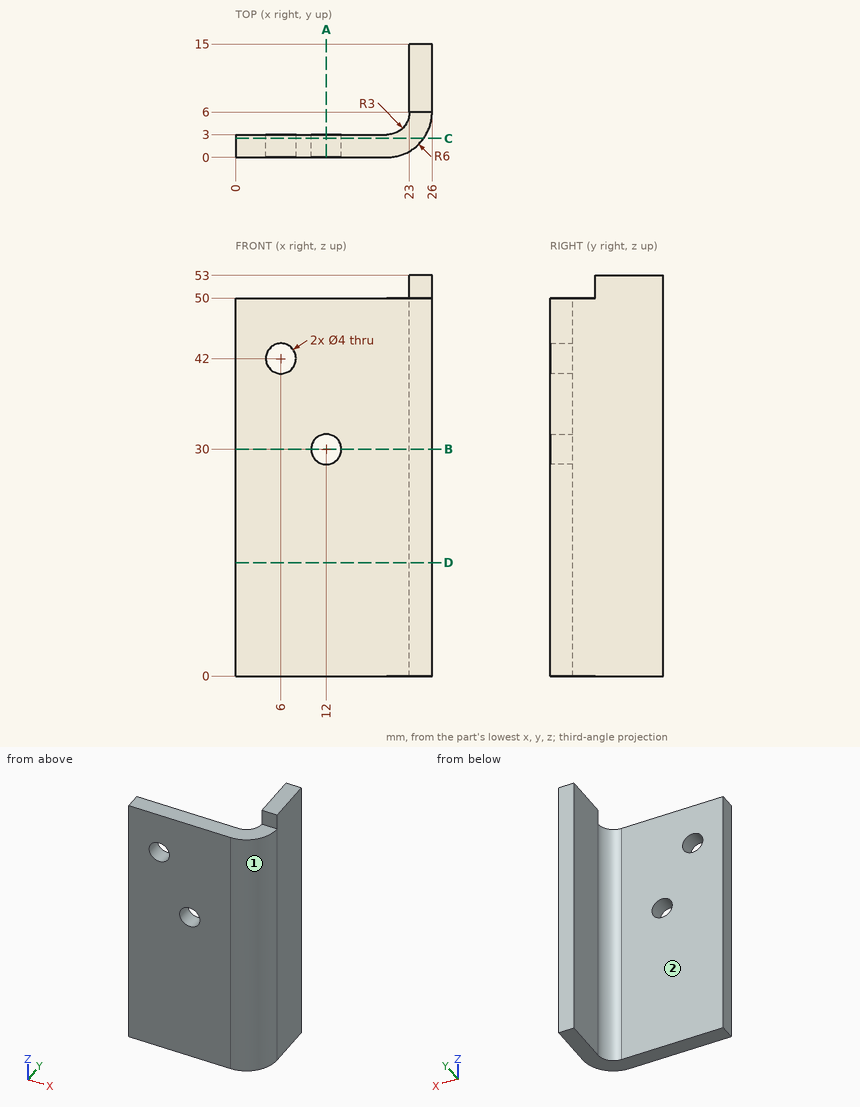
Design review of the part shown in the three views and the two pictorial views. Dimensions are in mm from the part's minimum x, y and z. A direction names the side the tool comes from. Give positions to 0.01 mm unless a question says otherwise; leave off trailing zeros. Loops run counter-clockwise (first coordinate to the right, second up) from the corner with the lowest first, then second, coordinate; pieces in that order, holes last. Notation, with made-up numbers: (52, 87) -> (88, 87) arc R10 ccw to (88, 92) -> close; hole circle Ø2 at (56.5, 10). An arc over 180 degrees is marked (long way). One line per question, with ' | ' between items.
1) To check wall thickness, follow probe 1 along X at (y, z) = (7.25, 39); probe 2 along Y at (x, z) = (4.5, 11.5); probe 3 along X at (y, z) = (0.7, 42). State the ranges of each line that lie inside material, in increasing order.
Resolved:
probe 1: x = 23 to 26 | probe 2: y = 0 to 3 | probe 3: x = 0 to 4, 8 to 22.81
2) We need section B-B (z = 30). Write out the cut boundary in (x, y).
Resolved:
outline: (0, 0) -> (10, 0) -> (10, 3) -> (0, 3) -> close; (14, 0) -> (20, 0) arc R6 ccw to (26, 6) -> (26, 15) -> (23, 15) -> (23, 6) arc R3 cw to (20, 3) -> (14, 3) -> close
3) We need section C-C (y = 2.5). Write out the cut boundary in (x, z).
Resolved:
outline: (0, 0) -> (24.87, 0) -> (24.87, 50) -> (0, 50) -> close; hole circle Ø4 at (6, 42); hole circle Ø4 at (12, 30)
4) We need section A-A (x = 12). Write out the cut boundary in (y, z), plus the area to 3 significant figures.
Resolved:
outline: (0, 0) -> (3, 0) -> (3, 28) -> (0, 28) -> close; (0, 32) -> (3, 32) -> (3, 50) -> (0, 50) -> close | area: 138 mm2
5) Insertion check: pin 1 Ø8 at (x, z) = (9, 21) entering from +Y; pin 2 Ø4 at (x, z) = (6, 39) entering from -Y; pin 3 Ø2.5 at (x, z) = (25, 51.5) entering from -Y; pin 4 Ø5 at (y, z) = (2, 33.5) entering from +X. Each pin has a flat end and moves straight along its axis. Give the tip position at first contact, or say it passes through.
Resolved:
pin 1: stops at y = 3 | pin 2: stops at y = 0 | pin 3: stops at y = 6 | pin 4: stops at x = 25.81
6) We need section D-D (z = 15). Write out the cut boundary in (x, y).
Resolved:
outline: (0, 0) -> (20, 0) arc R6 ccw to (26, 6) -> (26, 15) -> (23, 15) -> (23, 6) arc R3 cw to (20, 3) -> (0, 3) -> close
7) For the marked faces 1 and 2, list the 3-axis set-ups (+Z, -Z, +X, -X, +Y, -Y) from which the entire face can be reached by the end or side of a thin tool; tool diameter is ignored.
Resolved:
face 1: +Z, -Z, +X, -Y | face 2: +Z, -Z, -X, +Y
